Geometry check sheet. Reference: drawing and pictorial views, mm from the part's lowest x, y, z. Round coordinates to 2 decimals unless told otherwise and drop trailing zeros. Order: outer loops, then holes, each group sorted by start corner. A loop starts at its lowest first (then second) coordinate and runs counter-clockwise, first axis right, second up.
(1) Mould release check, pull along Z, two halves, no side actions. Record for the marked faces 1, 2 and 3: released by +Z, released by -Z, zero draft, split by the parting line, or undercut.
(2) Sectioned sample at D-D, the plane y = 20. Enter the section's corners in (x, z).
(3) Sectioned sample at C-C, the plane y = 12.7. Enter the section's corners in (x, z).
(4) Sectioned sample at B-B, the plane x = 50.8. Enter the section's corners in (y, z).
(5) Sectioned sample at A-A, the plane z = 50.8. Enter the section's corners in (x, y).
(6) Thickness scan on probe 1 along X at (y, z) = (12.7, 21); probe 2 along Z at (x, y) = (50.8, 17.5); probe 3 along X at (y, z) = (10.75, 86.5). Record the ranges inside material, lowest first.
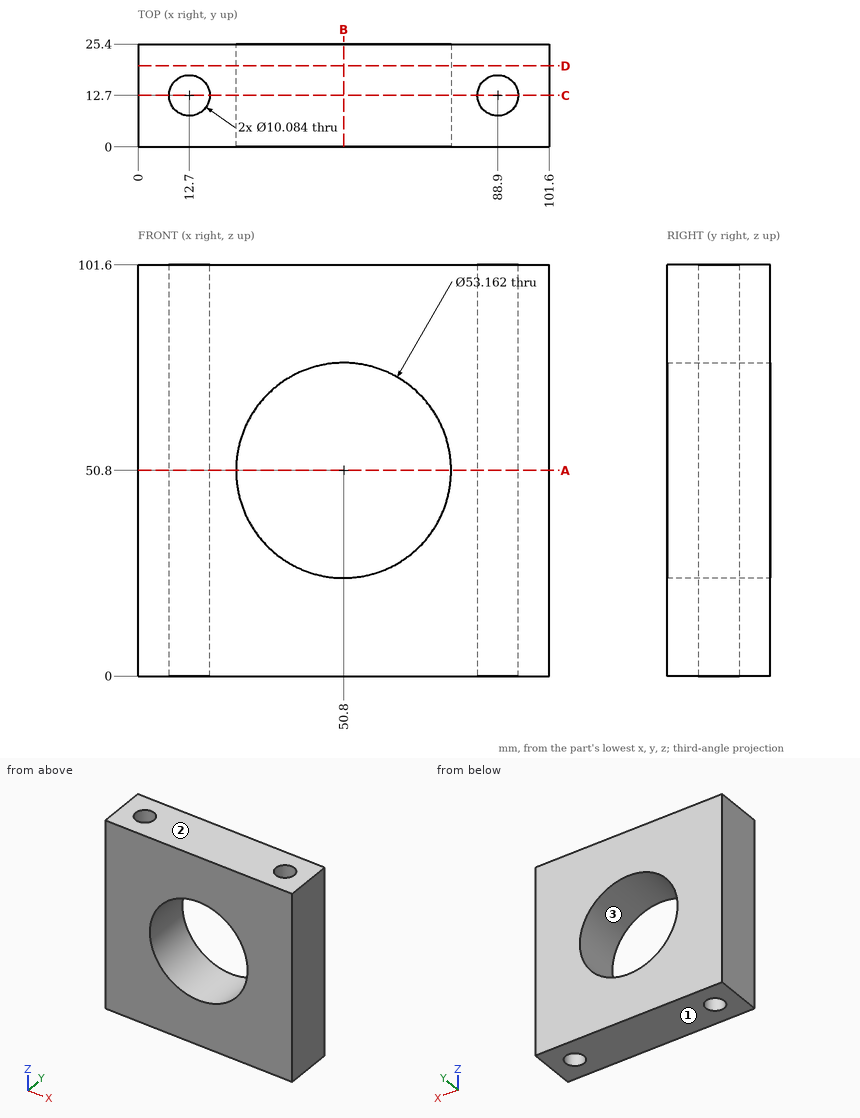
Derived:
1. face 1: released by -Z
1. face 2: released by +Z
1. face 3: undercut
2. outline: (0, 0) - (101.6, 0) - (101.6, 101.6) - (0, 101.6) - close; hole circle Ø53.16 at (50.8, 50.8)
3. outline: (0, 0) - (7.66, 0) - (7.66, 101.6) - (0, 101.6) - close; (17.74, 0) - (83.86, 0) - (83.86, 101.6) - (17.74, 101.6) - close; (93.94, 0) - (101.6, 0) - (101.6, 101.6) - (93.94, 101.6) - close; hole circle Ø53.16 at (50.8, 50.8)
4. outline: (0, 0) - (25.4, 0) - (25.4, 24.22) - (0, 24.22) - close; (0, 77.38) - (25.4, 77.38) - (25.4, 101.6) - (0, 101.6) - close
5. outline: (0, 0) - (24.22, 0) - (24.22, 25.4) - (0, 25.4) - close; (77.38, 0) - (101.6, 0) - (101.6, 25.4) - (77.38, 25.4) - close; hole circle Ø10.08 at (12.7, 12.7); hole circle Ø10.08 at (88.9, 12.7)
6. probe 1: x = 0 to 7.66, 17.74 to 83.86, 93.94 to 101.6
6. probe 2: z = 0 to 24.22, 77.38 to 101.6
6. probe 3: x = 0 to 8.05, 17.35 to 84.25, 93.55 to 101.6
